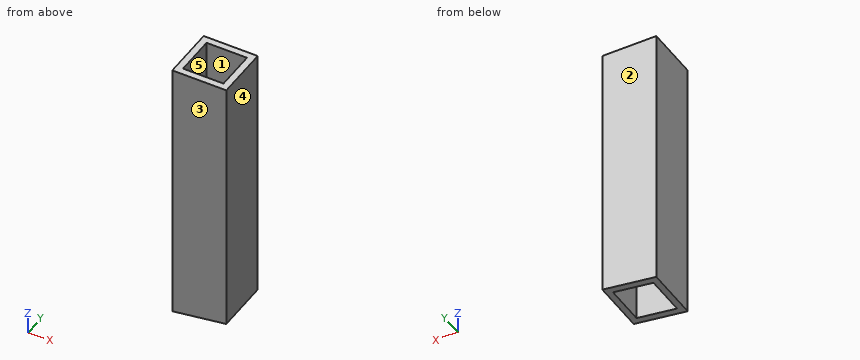
Autodesk Inventor part; units mm, degrees
ref_plane "YZ Plane" through (0, 0, 0) normal (1, 0, 0) x (0, 1, 0)
ref_plane "XZ Plane" through (0, 0, 0) normal (0, 1, 0) x (-1, 0, 0)
ref_plane "XY Plane" through (0, 0, 0) normal (0, 0, 1) x (1, 0, 0)
sketch "Sketch1" plane through (0, 0, 0) normal (0, 0, 1) x (1, 0, 0)
  line L0 (0, 0) -> (-25.4, 0)
  line L1 (-25.4, 0) -> (-25.4, 25.4)
  line L2 (-25.4, 25.4) -> (0, 25.4)
  line L3 (0, 25.4) -> (0, 0)
  line L4 (-3.175, 22.225) -> (-22.225, 22.225)
  line L5 (-22.225, 22.225) -> (-22.225, 3.175)
  line L6 (-22.225, 3.175) -> (-3.175, 3.175)
  line L7 (-3.175, 3.175) -> (-3.175, 22.225)
  dimension "d0" = 25.4
  dimension "d1" = 25.4
  dimension "d2" = 3.175
extrude "Extrusion1" add sketch "Sketch1" along normal blind 127
sketch "Sketch2" plane through (-25.4, 25.4, 0) normal (0, 1, 0) x (1, 0, 0)
  line L0 (0, 0) -> (25.4, 0)
  line L1 (25.4, 0) -> (25.4, -127)
  line L2 (0, 0) -> (25.4, -3.8097)
  dimension "d5" = 8.53
extrude "Extrusion2" cut sketch "Sketch2" against normal blind 127
Could you check a few things on this model? Use its own coordinates, in mm. Face numbers are marked on the shaded views. A direction names the side the tool comes from. Give positions to 0.01 mm unless a question says otherwise; leave off trailing zeros. Write each loop counter-clockwise with the first axis right and the second up, starting at its lowest first coordinate (ties: lowest second). Pieces come first, ordered by that corner, then holes. Notation, with made-up numbers: (-38.5, 2.25) -> (-2.5, 2.25) arc R22 ccw to (-2.5, 8.25) -> close; hole circle Ø1 at (-32, -21.75). An arc over 180 degrees is marked (long way). Answer as CSV lines item,"result". Start each with the question number.
(1) I'm going to push a flat-ended pin straight in: pin 1 Ø12 at (x, y) = (-16, 7.5) entering from -Z. Where does the tip first touch, or does it pass through?
(2) Please list where these lines run through material, in increasing order: line 1 (X direction, y = 20.5, z = 111.5) (3 decimals); line 2 (Y direction, x = -18.5, z = 65.5) (3 decimals); line 3 (Z direction, x = -23.5, y = 8.25).
(3) If we mould it in two halves opening along X, with no side actions, what happens to the marked faces 3, 4 and 5? For each: +X half, -X half, draft (parallel to the pull), parting line (faces both ways), or undercut.
(4) If we section it at B-B, the plane x = -17.75: Write out the boundary of the cut face in (y, z) (3 decimals), and give its area (3 significant figures).
(5) If we section it at C-C, the plane z = 46.5: Write out the boundary of the cut face in (x, y) (3 decimals).
(6) If we section it at A-A, the plane y = 10: Write out the boundary of the cut face in (x, z) (3 decimals).
(7) Which directions (+Z, -Z, +X, -X, +Y, -Y) give clear straight access to the entire face, cutting with the end or side of a thin tool? Please do the marked faces 1 and 2.
(8) If we section it at D-D, the plane x = -2: Write out the boundary of the cut face in (y, z).
Answer list:
1,pin 1,"z = 0.79"
2,line 1,"-25.4 to -22.225, -3.175 to 0"
2,line 2,"0 to 3.175, 22.225 to 25.4"
2,line 3,"0.28 to 127"
3,face 3,"draft"
3,face 4,"+X half"
3,face 5,"undercut"
4,outline,"(0, 1.147) -> (3.175, 1.147) -> (3.175, 127) -> (0, 127) -> close; (22.225, 1.147) -> (25.4, 1.147) -> (25.4, 127) -> (22.225, 127) -> close"
4,area,"799 mm^2"
5,outline,"(-25.4, 0) -> (0, 0) -> (0, 25.4) -> (-25.4, 25.4) -> close; hole (-22.225, 3.175) -> (-3.175, 3.175) -> (-3.175, 22.225) -> (-22.225, 22.225) -> close"
6,outline,"(-25.4, 0) -> (-22.225, 0.476) -> (-22.225, 127) -> (-25.4, 127) -> close; (-3.175, 3.333) -> (0, 3.81) -> (0, 127) -> (-3.175, 127) -> close"
7,face 1,"+Z, -Z"
7,face 2,"+Z, -Z, +X, -X, +Y"
8,outline,"(0, 3.51) -> (25.4, 3.51) -> (25.4, 127) -> (0, 127) -> close"
